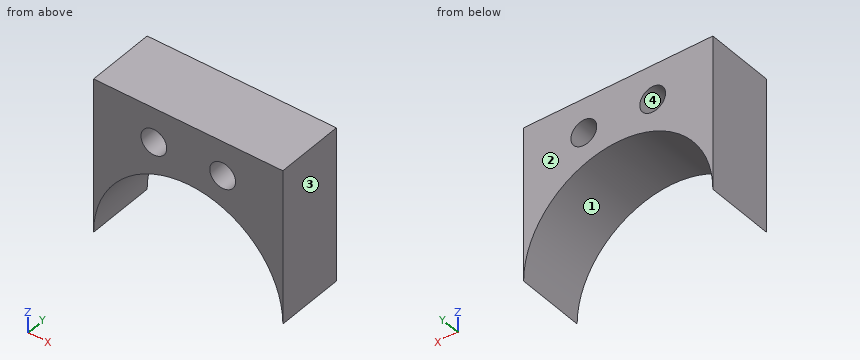
Autodesk Inventor part; units mm, degrees
ref_plane "YZ Plane" through (0, 0, 0) normal (1, 0, 0) x (0, 1, 0)
ref_plane "XZ Plane" through (0, 0, 0) normal (0, 1, 0) x (-1, 0, 0)
ref_plane "XY Plane" through (0, 0, 0) normal (0, 0, 1) x (1, 0, 0)
sketch "Boceto1" plane through (0, 0, 0) normal (0, 1, 0) x (-1, 0, 0)
  line L0 (0, 0) -> (-22, 0)
  line L1 (-22, 0) -> (-22, -18)
  line L2 (0, -18) -> (0, 0)
  arc A0 (0, -18) -> (-22, -18) centre (-11, -18) ccw
  circle A1 centre (-15, -4) radius 1.5
  circle A2 centre (-7, -4) radius 1.5
  dimension "d0" = 3
  dimension "d1" = 4
  dimension "d2" = 7
  dimension "d3" = 3
  dimension "d4" = 7
  dimension "d5" = 4
extrude "Extrusión1" add sketch "Boceto1" along normal blind 8
properties part number "CubreRodamiento" material "Nilón 6/6"
Design review of the part built by this model. Coordinates are the model's own, in mm. Face numbers are marked on the shaded views. Round coordinates to 2 decimals unless told otherwise and drop trailing zeros. Write each loop counter-clockwise with the first axis right and the second up, starting at its lowest first coordinate (ties: lowest second). Pieces come first, ordered by that corner, then holes.
Item 1: Wall thickness on L1, parallel to X at y = 3.25, z = -11; L2, parallel to Z at x = 11.25, y = 7.5; L3, parallel to Z at x = 7, y = 2: over which ranges is each line inside the solid? List them lowest first.
Item 2: Consider section A-A on z = -4. Give the boundary of the cut face in (x, y).
Item 3: Consider section C-C on y = 4.25. Give the boundary of the cut face in (x, z), and give its area (3 significant figures).
Item 4: Consider section B-B on x = 7. Give the boundary of the cut face in (y, z).
Item 5: Consider section D-D on z = -12. Give the boundary of the cut face in (x, y), and give its area (3 significant figures).
Item 6: For pin 1 Ø4 at (x, z) = (7, -4) entering from -Y, flat-tipped, find the tip position at first contact; note if it passes through.
Item 7: Draft analysis for pull direction X (two halves, no side actions). For the marked faces 1, 2, 3 and 4, state which applies: released by +X, released by -X, zero draft, split by the parting line, or undercut.
Check values:
1. L1: x = 0 to 2.51, 19.49 to 22
1. L2: z = -7 to 0
1. L3: z = -7.75 to -5.5, -2.5 to 0
2. outline: (0, 0) - (5.5, 0) - (5.5, 8) - (0, 8) - close; (8.5, 0) - (13.5, 0) - (13.5, 8) - (8.5, 8) - close; (16.5, 0) - (22, 0) - (22, 8) - (16.5, 8) - close
3. outline: (0, -18) arc R11 cw to (22, -18) - (22, 0) - (0, 0) - close; hole circle Ø3 at (7, -4); hole circle Ø3 at (15, -4)
3. area: 192 mm2
4. outline: (0, -7.75) - (8, -7.75) - (8, -5.5) - (0, -5.5) - close; (0, -2.5) - (8, -2.5) - (8, 0) - (0, 0) - close
5. outline: (0, 0) - (1.78, 0) - (1.78, 8) - (0, 8) - close; (20.22, 0) - (22, 0) - (22, 8) - (20.22, 8) - close
5. area: 28.5 mm2
6. pin 1: stops at y = 0
7. face 1: undercut
7. face 2: zero draft
7. face 3: released by +X
7. face 4: undercut
